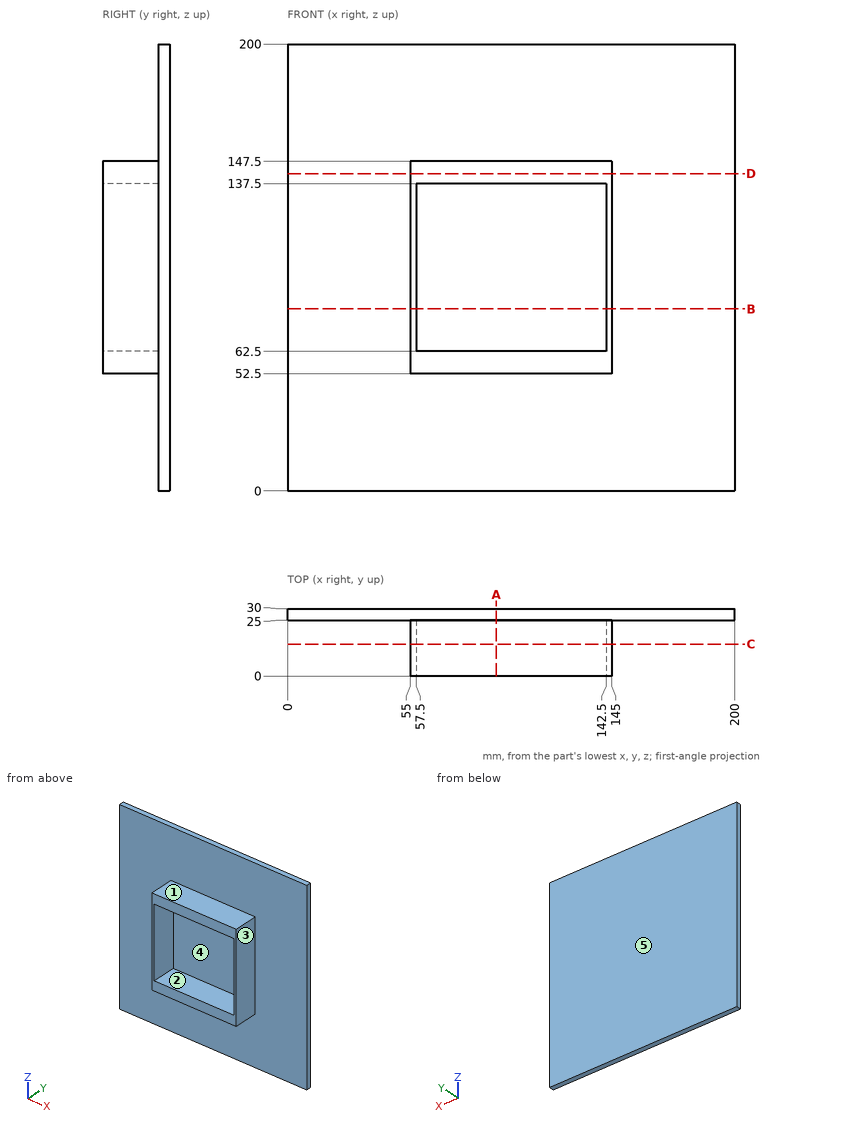
Could you check a few things on this drawing? It's one solid part, dimensions in mm from its lowest x, y, z. A direction names the side the tool comes from. Coordinates: 2 decimals unless noted, no trailing zeros. Loops run counter-clockwise (first coordinate to the right, second up) from the corner with the lowest first, then second, coordinate; pieces in that order, holes last. Notation, with made-up numbers: (11, -32) - (33, -32) arc R25 ccw to (33, -6) - close; hole circle Ø5 at (79.5, -27.5). An arc over 180 degrees is marked (long way). Answer as a JSON object with one key per item and string values. Group by question number.
Item 1: If we section it at D-D (z = 142): List the corners of the cut face in (x, y) for me.
Item 2: If we section it at C-C (y = 14.25): List the corners of the cut face in (x, z) for me, plus the area to 4 significant figures.
Item 3: If we section it at B-B (z = 81.5): List the corners of the cut face in (x, y) for me, plus the area to 4 significant figures.
Item 4: On a 3-axis mill with a long thin cutter (end or side, diameter ignored), from which of +Z, -Z, +X, -X, +Y, -Y can I reach the whole of each face in a straight line? I mean the marked faces 4 and 5. Say none if no direction works.
Item 5: For pin 1 (22.5 mm diameter, centred on x = 88, z = 84, fed in from -Y); pin 2 (7.5 mm diameter, centred on y = 17, z = 87, fed in from -X); pin 3 (10 mm diameter, centred on x = 53, y = 5, fed in from -Z), each with a flat end and sliding along its axis, tell me the tip position at first contact or that it passes through.
Item 6: If I drill on L1, parallel to X at y = 4.5, z = 73; L2, parallel to Z at x = 92, y = 6; L3, parallel to Y at x = 174.5, z = 159, over which ranges is the centre line in solid material (lowest first)? Write a range as from..to.
Item 7: If we section it at A-A (x = 93.5): List the corners of the cut face in (y, z) for me.
Item 8: If we mould it in two halves opening along Z, with no side actions, what happens to the marked faces 1, 2 and 3? For each: released by +Z, released by -Z, zero draft, split by the parting line, or undercut.
Returned:
{
 "1": {"outline": "(0, 25) - (55, 25) - (55, 0) - (145, 0) - (145, 25) - (200, 25) - (200, 30) - (0, 30) - close"},
 "2": {"outline": "(55, 52.5) - (145, 52.5) - (145, 147.5) - (55, 147.5) - close; hole (57.5, 62.5) - (142.5, 62.5) - (142.5, 137.5) - (57.5, 137.5) - close", "area": "2,175 mm²"},
 "3": {"outline": "(0, 25) - (55, 25) - (55, 0) - (57.5, 0) - (57.5, 25) - (142.5, 25) - (142.5, 0) - (145, 0) - (145, 25) - (200, 25) - (200, 30) - (0, 30) - close", "area": "1,125 mm²"},
 "4": {"face 4": "-Y", "face 5": "+Z, -Z, +X, -X, +Y"},
 "5": {"pin 1": "stops at y = 25", "pin 2": "stops at x = 55", "pin 3": "stops at z = 52.5"},
 "6": {"L1": "x = 55..57.5, 142.5..145", "L2": "z = 52.5..62.5, 137.5..147.5", "L3": "y = 25..30"},
 "7": {"outline": "(0, 52.5) - (25, 52.5) - (25, 0) - (30, 0) - (30, 200) - (25, 200) - (25, 147.5) - (0, 147.5) - (0, 137.5) - (25, 137.5) - (25, 62.5) - (0, 62.5) - close"},
 "8": {"face 1": "released by +Z", "face 2": "undercut", "face 3": "zero draft"}
}
